The listing builds one solid part. Answer for the finished solid, in the listing's coordinates (mm). Coordinates: 2 decimals unless noted, no trailing zeros. Loops run counter-clockwise (first coordinate to the right, second up) from the corner with the lowest first, then second, coordinate; pieces in that order, holes last. Notation, with made-up numbers: (-13, -8) - (38, -8) arc R21 ccw to (38, 3) - close; hole circle Ø11 at (15.25, -40). An arc over 180 degrees is marked (long way). Use one line per item in the form item = value. Start each with the question number.
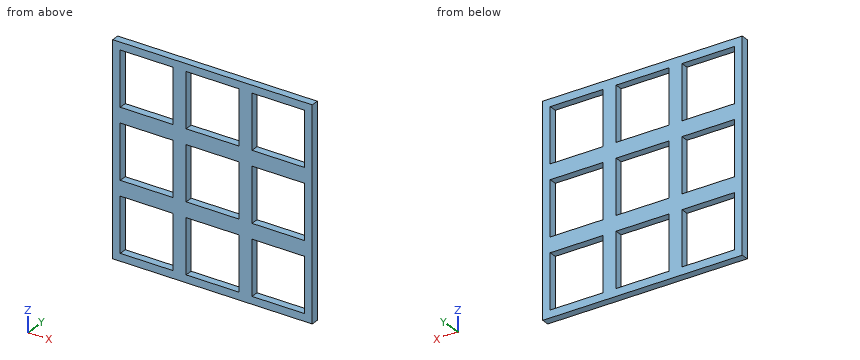
Autodesk Inventor part; units mm, degrees
ref_plane "YZ Plane" through (0, 0, 0) normal (1, 0, 0) x (0, 1, 0)
ref_plane "XZ Plane" through (0, 0, 0) normal (0, 1, 0) x (-1, 0, 0)
ref_plane "XY Plane" through (0, 0, 0) normal (0, 0, 1) x (1, 0, 0)
sketch "Sketch1" plane through (0, 0, 0) normal (0, 1, 0) x (-1, 0, 0)
  line L0 (-24.625, 24.95) -> (-24.625, -24.95)
  line L1 (24.625, 24.95) -> (-24.625, -24.95) construction
  line L2 (-24.625, 24.95) -> (24.625, -24.95) construction
  line L3 (-24.625, 22.95) -> (-22.625, 22.95) construction
  line L4 (-22.625, 24.95) -> (-22.625, 22.95) construction
  line L5 (-22.625, 22.95) -> (-8.575, 22.95)
  line L6 (-8.575, 22.95) -> (-8.575, 8.45)
  line L7 (-8.575, 8.45) -> (-22.625, 8.45)
  line L8 (-22.625, 8.45) -> (-22.625, 22.95)
  line L9 (-22.625, 8.45) -> (-22.625, 4.45) construction
  line L10 (-22.625, 4.45) -> (-8.575, 4.45)
  line L11 (-8.575, 4.45) -> (-8.575, -10.05)
  line L12 (-8.575, -10.05) -> (-22.625, -10.05)
  line L13 (-22.625, -10.05) -> (-22.625, 4.45)
  line L14 (-22.625, -10.05) -> (-22.625, -14.05) construction
  line L15 (-22.625, -14.05) -> (-8.575, -14.05)
  line L16 (-8.575, -14.05) -> (-8.575, -28.55)
  line L17 (-8.575, -28.55) -> (-22.625, -28.55)
  line L18 (-22.625, -28.55) -> (-22.625, -14.05)
  line L19 (-8.575, 22.95) -> (-5.075, 22.95) construction
  line L20 (-5.075, 22.95) -> (8.975, 22.95)
  line L21 (8.975, 22.95) -> (8.975, 8.45)
  line L22 (8.975, 8.45) -> (-5.075, 8.45)
  line L23 (-5.075, 8.45) -> (-5.075, 22.95)
  line L24 (-5.075, 8.45) -> (-5.075, 4.45)
  line L25 (-5.075, 4.45) -> (8.975, 4.45)
  line L26 (8.975, 4.45) -> (8.975, -10.05)
  line L27 (8.975, -10.05) -> (-5.075, -10.05)
  line L28 (-5.075, -10.05) -> (-5.075, 4.45)
  line L29 (-5.075, -10.05) -> (-5.075, -14.05) construction
  line L30 (-5.075, -14.05) -> (8.975, -14.05)
  line L31 (8.975, -14.05) -> (8.975, -28.55)
  line L32 (8.975, -28.55) -> (-5.075, -28.55)
  line L33 (-5.075, -28.55) -> (-5.075, -14.05)
  line L34 (8.975, 22.95) -> (12.475, 22.95) construction
  line L35 (12.475, 22.95) -> (26.525, 22.95)
  line L36 (26.525, 22.95) -> (26.525, 8.45)
  line L37 (26.525, 8.45) -> (12.475, 8.45)
  line L38 (12.475, 8.45) -> (12.475, 22.95)
  line L39 (8.975, 4.45) -> (12.475, 4.45) construction
  line L40 (12.475, 4.45) -> (26.525, 4.45)
  line L41 (26.525, 4.45) -> (26.525, -10.05)
  line L42 (26.525, -10.05) -> (12.475, -10.05)
  line L43 (12.475, -10.05) -> (12.475, 4.45)
  line L44 (12.475, -10.05) -> (12.475, -14.05) construction
  line L45 (12.475, -14.05) -> (26.525, -14.05)
  line L46 (26.525, -14.05) -> (26.525, -28.55)
  line L47 (26.525, -28.55) -> (12.475, -28.55)
  line L48 (12.475, -28.55) -> (12.475, -14.05)
  line L49 (-22.625, 24.95) -> (-24.625, 24.95)
  line L50 (-24.625, 24.95) -> (28.525, 24.95)
  line L51 (28.525, 24.95) -> (28.525, -30.55)
  line L52 (28.525, -30.55) -> (-24.625, -30.55)
  line L53 (-24.625, -30.55) -> (-24.625, 24.95)
  point P0 (0, 0)
  dimension "d3" = 2
  dimension "d4" = 14.5
  dimension "d5" = 14.05
  dimension "d6" = 4
  dimension "d7" = 14.5
  dimension "d8" = 14.05
  dimension "d9" = 4
  dimension "d10" = 14.5
  dimension "d11" = 14.05
  dimension "d12" = 2
  dimension "d13" = 3.5
  dimension "d14" = 14.5
  dimension "d15" = 14.05
  dimension "d16" = 4
  dimension "d17" = 14.5
  dimension "d18" = 14.05
  dimension "d19" = 4
  dimension "d20" = 14.5
  dimension "d21" = 3.5
  dimension "d22" = 14.05
  dimension "d23" = 3.5
  dimension "d24" = 14.5
  dimension "d25" = 4
  dimension "d26" = 14.5
  dimension "d27" = 55.5
  dimension "d28" = 53.15
  dimension "d29" = 14.05
  dimension "d32" = 14.5
extrude "Extrusion1" add sketch "Sketch1" along normal blind 2
properties part number "Keyframe3by3"
(1) This flat-tipped pin is pushed along its axis until it touches: pin 1 Ø1 at (x, z) = (-23, 2.5) entering from -Y. Where does it stop, or does it pass through?
(2) Find the intervals of material crossed by probe 1 along X at (y, z) = (0.2, 15.5) (3 decimals); probe 2 along Z at (x, y) = (1, 0.25), in increasing order. Write a range as from..to.
(3) A cutting plane is placed at A-A (x = -0.5). Determine the outline of the cut face in (y, z).
(4) A cutting plane is placed at C-C (y = 0.4). State how many separate pieces and enclosed holes the cut face has, then the cut area to 3 significant figures.
(5) A cutting plane is placed at B-B (z = -6). Determine the outline of the cut face in (x, y) (3 decimals).
Evaluation:
q1.pin_1 = through
q2.probe_1 = -28.525..-26.525, -12.475..-8.975, 5.075..8.575, 22.625..24.625
q2.probe_2 = -30.55..-28.55, -14.05..-10.05, 4.45..8.45, 22.95..24.95
q3.outline = (0, -30.55) - (2, -30.55) - (2, -28.55) - (0, -28.55) - close; (0, -14.05) - (2, -14.05) - (2, -10.05) - (0, -10.05) - close; (0, 4.45) - (2, 4.45) - (2, 8.45) - (0, 8.45) - close; (0, 22.95) - (2, 22.95) - (2, 24.95) - (0, 24.95) - close
q4.separate_pieces = 1
q4.enclosed_holes = 9
q4.area = 1,120 mm^2
q5.outline = (-28.525, 0) - (-26.525, 0) - (-26.525, 2) - (-28.525, 2) - close; (-12.475, 0) - (-8.975, 0) - (-8.975, 2) - (-12.475, 2) - close; (5.075, 0) - (8.575, 0) - (8.575, 2) - (5.075, 2) - close; (22.625, 0) - (24.625, 0) - (24.625, 2) - (22.625, 2) - close
